Can you work these out from the model? Positions are in its coordinate system, mm. Face numbers are marked on the shaded views. A direction names the side the tool comes from. Round coordinates to 2 decimals unless told otherwise and drop trailing zeros. Order: outer loops, then holes, each group sorted by start corner. A loop starts at its lowest first (then second) coordinate and runs counter-clockwise, first axis right, second up. Notation, with made-up numbers: (49.5, 68.25) -> (55.5, 68.25) arc R20 cw to (55.5, 74.25) -> close; hole circle Ø9 at (30, -23). An arc over 180 degrees is marked (long way). One line per item, written item: value.
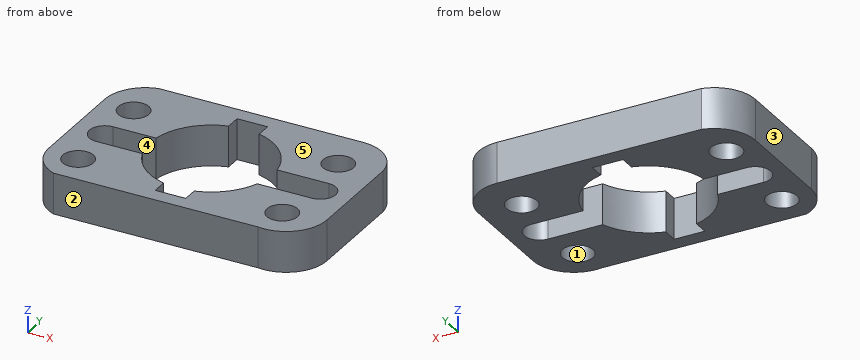
```python
from build123d import *

# Parameters (mm, degrees)
SKETCH1_R           = 9.525
BOSS_EXTRUDE1_DEPTH = 25.4


with BuildPart() as part:
    # Sketch1 → Boss-Extrude1 (new body)
    with BuildSketch(Plane.XY):
        with BuildLine():
            Line((-3.995852665, -20.577576414), (123.004147335, -20.577576414))
            ThreePointArc((123.004147335, -20.577576414), (143.432942762, -14.772522971), (152.311571269, 4.520073639))
            Line((152.311571269, 4.520073639), (152.311571269, 68.020073639))
            ThreePointArc((152.311571269, 68.020073639), (144.195614803, 84.596871175), (126.99997378, 91.302756331))
            Line((126.99997378, 91.302756331), (-2.622e-05, 91.302756331))
            ThreePointArc((-2.622e-05, 91.302756331), (-14.336851136, 82.409941414), (-19.939739045, 66.496602579))
            Line((-19.939739045, 66.496602579), (-19.939739045, 2.996602579))
            ThreePointArc((-19.939739045, 2.996602579), (-15.579526187, -11.233202656), (-3.995852665, -20.577576414))
        make_face()
        Circle(SKETCH1_R, mode=Mode.SUBTRACT)
        with Locations((0.00144481, 62.909901332)):
            Circle(SKETCH1_R, mode=Mode.SUBTRACT)
        with Locations((127.000131197, 63.487530849)):
            Circle(SKETCH1_R, mode=Mode.SUBTRACT)
        with Locations((126.999999388, -0.01246915)):
            Circle(SKETCH1_R, mode=Mode.SUBTRACT)
        with BuildLine():
            Line((-0.889739045, 41.26253085), (25.859586911, 41.26253085))
            ThreePointArc((25.859586911, 41.26253085), (35.282229592, 60.962735138), (53.975, 72.252756331))
            Line((53.975, 72.252756331), (53.975, 81.777756331))
            Line((53.975, 81.777756331), (62.356166676, 81.777756331))
            Line((62.356166676, 81.777756331), (73.025, 81.777756331))
            Line((73.025, 81.777756331), (73.025, 72.252756331))
            ThreePointArc((73.025, 72.252756331), (91.717770408, 60.962735138), (101.140413089, 41.26253085))
            Line((101.140413089, 41.26253085), (133.261571269, 41.26253085))
            ThreePointArc((133.261571269, 41.26253085), (142.786571269, 31.73753085), (133.261571269, 22.21253085))
            Line((133.261571269, 22.21253085), (99.258718454, 22.21253085))
            ThreePointArc((99.258718454, 22.21253085), (89.064662377, 7.11266894), (73.025, -1.527576414))
            Line((73.025, -1.527576414), (73.025, -11.052576414))
            Line((73.025, -11.052576414), (62.799638263, -11.052576414))
            Line((62.799638263, -11.052576414), (53.975, -11.052576414))
            Line((53.975, -11.052576414), (53.975, -1.527576414))
            ThreePointArc((53.975, -1.527576414), (37.935337623, 7.11266894), (27.741281546, 22.21253085))
            Line((27.741281546, 22.21253085), (-0.889739045, 22.21253085))
            ThreePointArc((-0.889739045, 22.21253085), (-10.414739045, 31.73753085), (-0.889739045, 41.26253085))
        make_face(mode=Mode.SUBTRACT)
    extrude(amount=BOSS_EXTRUDE1_DEPTH)


solid = part.part
```
Q1. I want a section at C-C on z = 2.25. List the corners of the cut face in (x, y) for me (3 decimals).
Answers below:
outline: (-19.94, 2.997) arc R25.4 ccw to (-3.996, -20.578) -> (123.004, -20.578) arc R25.4 ccw to (152.312, 4.52) -> (152.312, 68.02) arc R25.4 ccw to (127, 91.303) -> (0, 91.303) arc R25.4 ccw to (-19.94, 66.497) -> close; hole circle Ø19.05 at (0, 0); hole circle Ø19.05 at (0.001, 62.91); hole (-0.89, 22.213) -> (27.741, 22.213) arc R38.1 ccw to (53.975, -1.528) -> (53.975, -11.053) -> (73.025, -11.053) -> (73.025, -1.528) arc R38.1 ccw to (99.259, 22.213) -> (133.262, 22.213) arc R9.525 ccw to (133.262, 41.263) -> (101.14, 41.263) arc R38.1 ccw to (73.025, 72.253) -> (73.025, 81.778) -> (53.975, 81.778) -> (53.975, 72.253) arc R38.1 ccw to (25.86, 41.263) -> (-0.89, 41.263) arc R9.525 ccw to start; hole circle Ø19.05 at (127, -0.012); hole circle Ø19.05 at (127, 63.488)
Q2. On a 3-axis mill with a long thin cutter (end or side, diameter ignored), from which of +Z, -Z, +X, -X, +Y, -Y can I reach the whole of each face in a straight line? I mean the marked faces 4 and 5. Say none if no direction works.
Answers below:
face 4: +Z, -Z
face 5: +Z, +X, -X, +Y, -Y
Q3. I want a section at D-D on y = -4. List the corners of the cut face in (x, z) for me (3 decimals).
Answers below:
outline: (-18.957, 0) -> (-8.644, 0) -> (-8.644, 25.4) -> (-18.957, 25.4) -> close; (8.644, 0) -> (53.975, 0) -> (53.975, 25.4) -> (8.644, 25.4) -> close; (73.025, 0) -> (118.35, 0) -> (118.35, 25.4) -> (73.025, 25.4) -> close; (135.65, 0) -> (150.84, 0) -> (150.84, 25.4) -> (135.65, 25.4) -> close
Q4. We'd pull the mould along X, two halves only. Please class the marked faces 1, 2 and 3: released by +X, released by -X, zero draft, split by the parting line, or undercut.
Answers below:
face 1: undercut
face 2: zero draft
face 3: released by -X
Q5. Please list where these lines run through material, in increasing order: line 1 along Y through (x, z) = (127, 11); line 2 along Y through (x, z) = (123, 4.75); line 3 along X through (y, z) = (69, 21).
Answers below:
line 1: -20.88 to -9.54, 9.51 to 22.21, 41.26 to 53.96, 73.01 to 91.3
line 2: -20.58 to -8.66, 8.63 to 22.21, 41.26 to 54.84, 72.13 to 91.3
line 3: -19.82 to -7.32, 7.33 to 45.61, 81.39 to 119.23, 134.77 to 152.21
Q6. I want a section at B-B on y = 70. List the corners of the cut face in (x, z) for me.
Answers below:
outline: (-19.7, 0) -> (-6.36, 0) -> (-6.36, 25.4) -> (-19.7, 25.4) -> close; (6.36, 0) -> (47.63, 0) -> (47.63, 25.4) -> (6.36, 25.4) -> close; (79.37, 0) -> (120.05, 0) -> (120.05, 25.4) -> (79.37, 25.4) -> close; (133.95, 0) -> (152.07, 0) -> (152.07, 25.4) -> (133.95, 25.4) -> close
Q7. Will these pins go through, and if not, where does the flat tip stop? pin 1 Ø5 at (y, z) = (78, 9) entering from +X; pin 2 Ø1.5 at (x, y) = (94, 4) entering from -Z; pin 3 Ø10.5 at (y, z) = (75.5, 15) entering from -X; pin 4 Ø5 at (y, z) = (-5.5, 7.5) entering from -X.
Answers below:
pin 1: x = 150.52
pin 2: z = 0
pin 3: x = -19.66
pin 4: x = -19.22
Q8. I want a section at A-A on x = 103. List the corners of the cut face in (y, z) for me, plus the area to 3 significant figures.
Answers below:
outline: (-20.58, 0) -> (22.21, 0) -> (22.21, 25.4) -> (-20.58, 25.4) -> close; (41.26, 0) -> (91.3, 0) -> (91.3, 25.4) -> (41.26, 25.4) -> close
area: 2,360 mm^2
